Build history of the part. All positions in model axes, mm. A direction names the side the tool comes from. Round coordinates to 2 decimals unless told otherwise and drop trailing zeros. Loops run counter-clockwise (first coordinate to the right, second up) from the corner with the lowest first, then second, coordinate; pieces in that order, holes last. Notation, with made-up numbers: (21.5, 82.5) - (40.5, 82.5) arc R27 ccw to (40.5, 114.5) - close; hole circle Ø11 at (26, 62.5). An arc over 180 degrees is marked (long way). Use a Markdown table: item, result.
from build123d import *

# Parameters (mm, degrees)
F0_W          = 6
F0_H          = 6
F1_DEPTH      = 3.6
F2_R          = 1.8
F3_DEPTH      = 0.7
F4_W          = 0.35
F4_H          = 0.7
F5_DEPTH      = 1
F5_DEPTH_BACK = 7


with BuildPart() as f1:
    # F0 (on Front) → F1 (new body)
    with BuildSketch(Plane.XZ):
        with Locations((-54.375002, 35.616073)):
            Rectangle(F0_W, F0_H)
    extrude(amount=F1_DEPTH)

    # F2 (on face) → F3 (join)
    with BuildSketch(Plane.XZ.offset(3.6)):
        with Locations((-54.375002, 35.616073)):
            Circle(F2_R)
    extrude(amount=F3_DEPTH)

    # F4 (on face) → F5 (join, two sides)
    with BuildSketch(Plane(origin=(-57.375002, 0, 0), x_dir=(0, -1, 0), z_dir=(-1, 0, 0))) as f5_sk:
        with Locations((0.175, 37.866073)):
            Rectangle(F4_W, F4_H)
        with Locations((0.175, 33.366073)):
            Rectangle(F4_W, F4_H)
    extrude(amount=F5_DEPTH)
    extrude(f5_sk.sketch, amount=-F5_DEPTH_BACK)


solid = f1.part
Q1. Cut at B-B, the plane z = 36.9. List the corners of the cut face in (x, y) (3 decimals), plus the area to 3 significant figures.
Results found:
| item | result |
|---|---|
| outline | (-57.375, -3.6) - (-55.637, -3.6) - (-55.637, -4.3) - (-53.113, -4.3) - (-53.113, -3.6) - (-51.375, -3.6) - (-51.375, 0) - (-57.375, 0) - close |
| area | 23.4 mm2 |
Q2. Cut at C-C, the plane y = -1.4. List the corners of the cut face in (x, z) (3 decimals), plus the area to 3 significant figures.
Results found:
| item | result |
|---|---|
| outline | (-57.375, 32.616) - (-51.375, 32.616) - (-51.375, 38.616) - (-57.375, 38.616) - close |
| area | 36.0 mm2 |
Q3. Cut at A-A, the plane x = -50.75. List the corners of the cut face in (y, z).
Results found:
| item | result |
|---|---|
| outline | (-0.35, 33.02) - (0, 33.02) - (0, 33.72) - (-0.35, 33.72) - close; (-0.35, 37.52) - (0, 37.52) - (0, 38.22) - (-0.35, 38.22) - close |
Q4. Drop flat-ended pins along their axis: pin 1 (0.6 mm diameter, centred on x = -58, z = 37.5, fed in from -Y); pin 2 (2 mm diameter, centred on x = -57, z = 34, fed in from +Y); pin 3 (1 mm diameter, centred on x = -57, z = 36.5, fed in from -Y); pin 4 (1.5 mm diameter, centred on y = -3, z = 37.5, fed in from +X) (3 decimals). Give the stop position or say it passes through.
Results found:
| item | result |
|---|---|
| pin 1 | stops at y = -0.35 |
| pin 2 | stops at y = 0 |
| pin 3 | stops at y = -3.6 |
| pin 4 | stops at x = -51.375 |
Q5. Which spindle directions (+Z, -Z, +X, -X, +Y, -Y) get a long thin tool onto all of the face, cutting with end or side? Do faces 1 (the face through (-56, -3.6, 34)), 2 (the face through (-54, -2, 32.616)). Say none if no direction does.
Results found:
| item | result |
|---|---|
| face 1 | -Y |
| face 2 | -Z, +X, -X, +Y, -Y |
Q6. Cut at D-D, the plane x = -55. List the corners of the cut face in (y, z), plus the area to 3 significant figures.
Results found:
| item | result |
|---|---|
| outline | (-4.3, 33.93) - (-3.6, 33.93) - (-3.6, 32.62) - (0, 32.62) - (0, 38.62) - (-3.6, 38.62) - (-3.6, 37.3) - (-4.3, 37.3) - close |
| area | 24.0 mm2 |
Q7. Probe line 1 (X direction, y = -3, z = 35.95) (3 decimals); line 2 (Y direction, x = -52.75, z = 34.55); line 3 (Y direction, x = -50.75, z = 33.15). List the from-to ranges inside material, lowest first.
Results found:
| item | result |
|---|---|
| line 1 | x = -57.375 to -51.375 |
| line 2 | y = -3.6 to 0 |
| line 3 | y = -0.35 to 0 |
